Geometry: final body of the model. Coordinates: model frame, mm. Face numbers are marked on the shaded views. A direction names the side the tool comes from. Give positions to 0.01 mm unless a question says otherwise; leave off trailing zeros. Write each loop counter-clockwise with the first axis right and the second up, starting at its lowest first coordinate (ties: lowest second). Pieces come first, ordered by that corner, then holes.
Q1. Line query: line 1 (X direction, y = -23.5, z = 3.25); line 2 (X direction, y = -11.75, z = 3.4); line 3 (Y direction, x = 12.75, z = 3.85). Output: solid intervals per line, ascending.
Q2. Section A-A (x = 29.5). Return the cut outline in (y, z).
Q3. Section D-D (z = 3.45). Return the cut outline in (x, y) (3 decimals), plus the area to 3 significant figures.
Q4. Reachability of the marked faces 1 and 2 from +Z, -Z, +X, -X, +Y, -Y: full face, straight path, thin tool, end or side. Return the list, or none.
Q5. Section B-B (y = -2.5). Return the cut outline in (x, z), plus the area to 3 significant figures.
Q6. Section C-C (y = 0.75). Return the cut outline in (x, z).
Q7. Pin query (flat end, axial travel): pin 1 Ø1.9 at (x, y) = (36.99, -23.63) entering from +Z; pin 2 Ø4 at (x, y) = (12.99, 0.37) entering from -Z; pin 3 Ø2 at (x, z) = (27, 1) entering from -Y. Return the tip coordinate at first contact, or that it passes through.
from build123d import *

# Parameters (mm, degrees)
ESQUISSE1_R             = 13.75
ESQUISSE1_R_2           = 10.75
BOSS_EXTRU_1_DEPTH      = 2.5
ESQUISSE2_W             = 30
ESQUISSE2_H             = 30
ESQUISSE2_R             = 1.625
BOSS_EXTRU_2_DEPTH      = 2
ESQUISSE3_R             = 10.75
ENL_V_MAT_EXTRU_1_DEPTH = 23
CONG_1_R                = 1


with BuildPart() as part:
    # Esquisse1 → Boss.-Extru.1 (new body)
    with BuildSketch(Plane.XY):
        with Locations((24.994563159, -11.631436553)):
            Circle(ESQUISSE1_R)
        with Locations((24.994563159, -11.631436553)):
            Circle(ESQUISSE1_R_2, mode=Mode.SUBTRACT)
    extrude(amount=BOSS_EXTRU_1_DEPTH)

    # Esquisse2 → Boss.-Extru.2 (add)
    with BuildSketch(Plane.XY.offset(2.5)):
        with Locations((24.994563159, -11.631436553)):
            Rectangle(ESQUISSE2_W, ESQUISSE2_H)
        with Locations((12.994563159, 0.368563447)):
            Circle(ESQUISSE2_R, mode=Mode.SUBTRACT)
        with Locations((36.994563159, 0.368563447)):
            Circle(ESQUISSE2_R, mode=Mode.SUBTRACT)
        with Locations((12.994563159, -23.631436553)):
            Circle(ESQUISSE2_R, mode=Mode.SUBTRACT)
        with Locations((36.994563159, -23.631436553)):
            Circle(ESQUISSE2_R, mode=Mode.SUBTRACT)
    extrude(amount=BOSS_EXTRU_2_DEPTH)

    # Esquisse3 → Enlèv. mat.-Extru.1 (cut)
    with BuildSketch(Plane(origin=(0, 0, 0), x_dir=(-1, 0, 0), z_dir=(0, 0, -1))):
        with Locations((-24.994563159, -11.631436553)):
            Circle(ESQUISSE3_R)
    extrude(amount=-ENL_V_MAT_EXTRU_1_DEPTH, mode=Mode.SUBTRACT)

    # Congé1
    cong_1_edges = [part.edges().sort_by_distance(p)[0] for p in [
        (9.994563159, 3.368563447, 3.5),
        (9.994563159, -26.631436553, 3.5),
        (39.994563159, -26.631436553, 3.5),
        (39.994563159, 3.368563447, 3.5),
    ]]
    fillet(cong_1_edges, radius=CONG_1_R)


solid = part.part
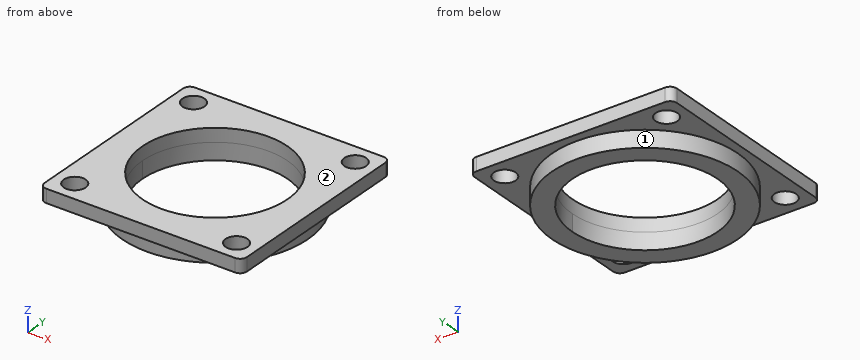
Computed:
1. line 1: x = 9.99 to 11.37, 14.61 to 35.37, 38.61 to 39.99
1. line 2: x = 9.99 to 14.25, 35.74 to 39.99
1. line 3: y = -26.63 to -25.24, -22.02 to -1.24, 1.98 to 3.37
2. outline: (-26.63, 2.5) - (-24.62, 2.5) - (-24.62, 0) - (-21.39, 0) - (-21.39, 4.5) - (-26.63, 4.5) - close; (-1.87, 0) - (1.36, 0) - (1.36, 2.5) - (3.37, 2.5) - (3.37, 4.5) - (-1.87, 4.5) - close
3. outline: (9.995, -25.631) arc R1 ccw to (10.995, -26.631) - (38.995, -26.631) arc R1 ccw to (39.995, -25.631) - (39.995, 2.369) arc R1 ccw to (38.995, 3.369) - (10.995, 3.369) arc R1 ccw to (9.995, 2.369) - close; hole circle Ø3.25 at (12.995, -23.631); hole circle Ø3.25 at (12.995, 0.369); hole circle Ø21.5 at (24.995, -11.631); hole circle Ø3.25 at (36.995, -23.631); hole circle Ø3.25 at (36.995, 0.369)
3. area: 503 mm2
4. face 1: -Z
4. face 2: +Z, +X, -X, +Y, -Y
5. outline: (9.99, 2.5) - (14.71, 2.5) - (14.71, 0) - (19.32, 0) - (19.32, 4.5) - (9.99, 4.5) - close; (30.67, 0) - (35.27, 0) - (35.27, 2.5) - (39.99, 2.5) - (39.99, 4.5) - (30.67, 4.5) - close
5. area: 60.3 mm2
6. outline: (9.99, 2.5) - (11.41, 2.5) - (11.41, 4.5) - (9.99, 4.5) - close; (14.57, 2.5) - (19.01, 2.5) - (19.01, 0) - (30.97, 0) - (30.97, 2.5) - (35.41, 2.5) - (35.41, 4.5) - (14.57, 4.5) - close; (38.57, 2.5) - (39.99, 2.5) - (39.99, 4.5) - (38.57, 4.5) - close
7. pin 1: passes through
7. pin 2: stops at z = 2.5
7. pin 3: stops at y = -25.34
